Could you check a few things on this drawing? It's one solid part, dimensions in mm from its lowest x, y, z. A direction names the side the tool comes from. Coordinates: 2 decimals unless noted, no trailing zeros. Loops run counter-clockwise (first coordinate to the right, second up) from the corner with the lowest first, then second, coordinate; pieces in that order, holes last. Notation, with made-up numbers: M -10,20 L 42,20 A19 cw 42,42 Z; hole C 86,3 d2. An arc over 180 degrees is marked long. Answer as a JSON object with one key per item and string values. Group by question number.
Item 1: Suppose I cut it at A-A (y = 4). Write out the boundary of the cut face in (x, z).
Item 2: Which directions (+Z, -Z, +X, -X, +Y, -Y) give clear straight access to the entire face, cutting with the end or side of a thin tool? Please do the marked faces 1, 2 and 3.
Item 3: I'm going to push flat-ended pins straight in: pin 1 Ø1.5 at (x, z) = (2.5, 22.5) entering from -Y; pin 2 Ø1 at (x, z) = (4.5, 15.5) entering from +Y (1 decimal); pin 3 Ø1 at (y, z) = (4, 7.5) entering from +X. Where does each tip first touch, or does it pass through?
Item 4: Suppose I cut it at B-B (z = 14). Write out the boundary of the cut face in (x, y) (1 decimal).
Item 5: Suppose I cut it at C-C (x = 0.5). Write out the boundary of the cut face in (y, z).
Item 6: Suppose I cut it at D-D (y = 5.75). Write out the boundary of the cut face in (x, z), then the cut area to 3 significant figures.
Item 7: If I drill on line 1 (Z direction, x = 5, y = 1.25); line 2 (Y direction, x = 3.25, z = 20) (1 decimal); line 3 (X direction, y = 1.25, z = 26.5) (1 decimal), over which ranges is the centre line in solid material (lowest first)?
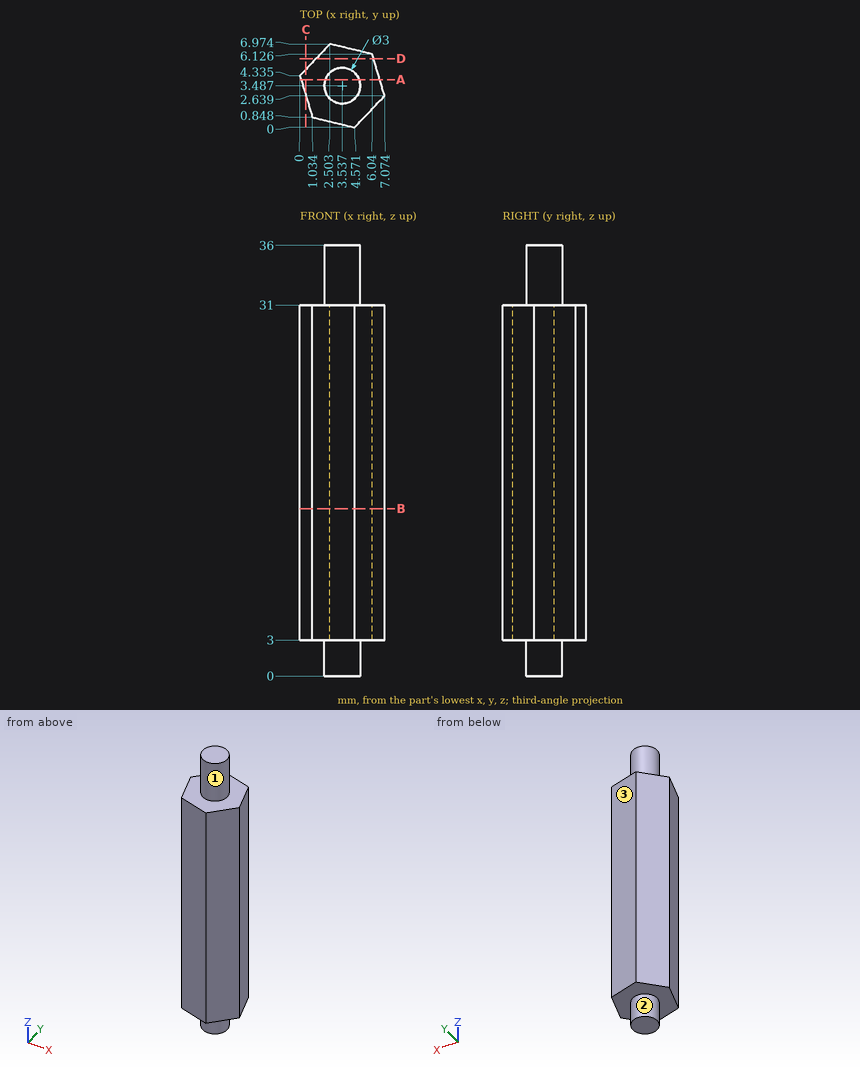
From the geometry:
{
 "1": {"outline": "M 0.1,3 L 2.13,3 L 2.13,0 L 4.95,0 L 4.95,3 L 6.67,3 L 6.67,31 L 4.95,31 L 4.95,36 L 2.13,36 L 2.13,31 L 0.1,31 Z"},
 "2": {"face 1": "+Z", "face 2": "-Z", "face 3": "+Z, -Z, +X, +Y"},
 "3": {"pin 1": "y = 0.32", "pin 2": "y = 6.6", "pin 3": "x = 6.82"},
 "4": {"outline": "M 0,4.3 L 1,0.8 L 4.6,0 L 7.1,2.6 L 6,6.1 L 2.5,7 Z"},
 "5": {"outline": "M 2.65,3 L 4.86,3 L 4.86,31 L 2.65,31 Z"},
 "6": {"outline": "M 1.34,3 L 6.15,3 L 6.15,31 L 1.34,31 Z", "area": "135 mm2"},
 "7": {"line 1": "3 to 31", "line 2": "0.3 to 6.8", "line 3": "0.9 to 5.8"}
}
